Build history of the part. All positions in model axes, mm. A direction names the side the tool comes from. Round coordinates to 2 decimals unless told otherwise and drop trailing zeros. Write each loop counter-clockwise with the first axis right and the second up, starting at its lowest first coordinate (ties: lowest second). Pieces come first, ordered by that corner, then holes. Notation, with made-up numbers: (-1.5, 20) - (27.5, 20) arc R7 cw to (27.5, 33) - close; hole circle Ø7 at (-21, 39.5). An arc over 180 degrees is marked (long way). Answer as a JSON object with one key per item and string values. Group by question number.
Item 1: Which spindle directions (+Z, -Z, +X, -X, +Y, -Y) get a long thin tool onto all of the face, cutting with end or side? Do faces 1 (the flat face through (13.52, 5.77, 41.77)), 2 (the flat face through (7.254, 4.056, -15.687)), 3 (the cylindrical face through (9.31, 7.43, -43.15)). Say none if no direction does.
Item 2: Slice it at D-D, the plane z = -38.75. List the corners of the cut face in (x, y).
Item 3: Two-plate mould, pull along X, no slides. Class faces 4 (the cylindrical face through (9, 4, 41)), 5 (the flat face through (14.3, 7.2, -0.6)), 6 (the flat face through (10.032, 4, 10)), 7 (the flat face through (-14.26, 3.97, -42.99)): +X half, -X half, draft (parallel to the pull), parting line (faces both ways), or undercut.
Item 4: Flat gauge pins, fed straight in: pin 1 (3.5 mm diameter, centred on y = 4, z = 38.75, fed in from -X) (3 decimals); pin 2 (2.5 mm diameter, centred on x = -2.5, y = 5, fed in from +Z). Where does each tip first touch, or does it go through?
Item 5: Probe line 1 (Y direction, x = 8.5, z = -38.75); line 2 (Y direction, x = 12.25, z = 40.5); line 3 (X direction, y = 4.25, z = -13.5). List the from-to ranges inside material, lowest first. Write a range as from..to.
Item 6: Slice it at B-B, the plane x = -7. List the corners of the cut face in (y, z).
Item 7: Slice it at A-A, the plane z = 38.75. List the corners of the cut face in (x, y).
Item 8: Slice it at C-C, the plane x = -12.25. List the corners of the cut face in (y, z).
from build123d import *

# Parameters (mm, degrees)
SKETCH1_W           = 30
SKETCH1_H           = 87.5
BOSS_EXTRUDE1_DEPTH = 8
SKETCH2_W           = 10
SKETCH2_H           = 12
CUT_EXTRUDE1_DEPTH  = 8
SKETCH3_R           = 2.25
CUT_EXTRUDE2_DEPTH  = 54.647576833
FILLET1_R           = 2
CUT_EXTRUDE3_DEPTH  = 47.936792605
FILLET2_R           = 3
CHAMFER1_SIZE       = 1.5
FILLET3_R           = 0.5
CUT_EXTRUDE4_DEPTH  = 3


with BuildPart() as part:
    # Sketch1 → Boss-Extrude1 (new body)
    with BuildSketch(Plane(origin=(0, 0, 0), x_dir=(1, 0, 0), z_dir=(0, 1, 0))):
        Rectangle(SKETCH1_W, SKETCH1_H)
    extrude(amount=BOSS_EXTRUDE1_DEPTH)

    # Sketch2 → Cut-Extrude1 (cut)
    with BuildSketch(Plane(origin=(0, 8, 0), x_dir=(1, 0, 0), z_dir=(0, 1, 0))):
        with Locations((0, 37.75)):
            Rectangle(SKETCH2_W, SKETCH2_H)
        with Locations((0, -37.75)):
            Rectangle(SKETCH2_W, SKETCH2_H)
    extrude(amount=-CUT_EXTRUDE1_DEPTH, mode=Mode.SUBTRACT)

    # Sketch3 → Cut-Extrude2 (cut, through all)
    with BuildSketch(Plane(origin=(15, 0, 0), x_dir=(0, 0, -1), z_dir=(1, 0, 0))):
        with Locations((-38.75, 4)):
            Circle(SKETCH3_R)
    cut_extrude2 = extrude(amount=-CUT_EXTRUDE2_DEPTH, mode=Mode.SUBTRACT)

    # Mirror1: Cut-Extrude2 across plane
    add(cut_extrude2.mirror(Plane.XY), mode=Mode.SUBTRACT)

    # Fillet1
    fillet1_edges = [part.edges().sort_by_distance(p)[0] for p in [
        (10, 0, 43.75),
        (-10, 0, -43.75),
        (-10, 8, 43.75),
        (-10, 8, -43.75),
        (10, 8, 43.75),
        (-10, 0, 43.75),
        (10, 0, -43.75),
        (10, 8, -43.75),
    ]]
    fillet(fillet1_edges, radius=FILLET1_R)

    # Sketch4 → Cut-Extrude3 (cut, through all)
    with BuildSketch(Plane(origin=(0, 8, 0), x_dir=(1, 0, 0), z_dir=(0, 1, 0))):
        Polygon((5, 24.75), (-10, 24.75), (1.511627907, 13.238372093), align=None)
        Polygon((10, 4.75), (10, 24.75), (5.348837209, 9.401162791), align=None)
        Polygon((-10, -4.75), (-10, -24.75), (-5.348837209, -9.401162791), align=None)
        Polygon((-5, -24.75), (10, -24.75), (-1.511627907, -13.238372093), align=None)
        Polygon((-10, 17.678932188), (-10, 2.321067812), (-3.704402834, -3.974529354), (-0.132806468, 7.811738656), align=None)
        Polygon((10.032301404, -17.711233593), (10.032301404, -2.353369216), (3.704402834, 3.974529354), (0.132806468, -7.811738656), align=None)
    extrude(amount=-CUT_EXTRUDE3_DEPTH, mode=Mode.SUBTRACT)

    # Fillet2
    fillet2_edges = [part.edges().sort_by_distance(p)[0] for p in [
        (0, 0, -31.75),
        (0, 0, 31.75),
    ]]
    fillet(fillet2_edges, radius=FILLET2_R)

    # Chamfer1
    chamfer1_edges = [part.edges().sort_by_distance(p)[0] for p in [
        (15, 4, -43.75),
        (15, 0, 0),
        (-15, 0, 0),
        (15, 8, 0),
        (15, 4, 43.75),
        (15, 7.414213562, 43.164213562),
        (15, 0.585786438, 43.164213562),
        (15, 7.414213562, -43.164213562),
        (15, 0.585786438, -43.164213562),
        (-15, 8, 0),
        (-15, 4, 43.75),
        (-15, 4, -43.75),
        (-15, 0.585786438, 43.164213562),
        (-15, 7.414213562, 43.164213562),
        (-15, 0.585786438, -43.164213562),
        (-15, 7.414213562, -43.164213562),
    ]]
    chamfer(chamfer1_edges, length=CHAMFER1_SIZE)

    # Fillet3
    fillet3_edges = [part.edges().sort_by_distance(p)[0] for p in [
        (-10, 4, -17.678932188),
        (-0.132806468, 4, -7.811738656),
        (-3.704402834, 4, 3.974529354),
        (-10, 4, -2.321067812),
        (-1.511627907, 4, 13.238372093),
        (10, 4, 24.75),
        (-5, 4, 24.75),
        (10, 4, -4.75),
        (5.348837209, 4, -9.401162791),
        (10, 4, -24.75),
        (-10, 4, 4.75),
        (-5.348837209, 4, 9.401162791),
        (-10, 4, 24.75),
        (10.032301404, 4, 17.711233593),
        (0.132806468, 4, 7.811738656),
        (3.704402834, 4, -3.974529354),
        (10.032301404, 4, 2.353369216),
        (5, 4, -24.75),
        (1.511627907, 4, -13.238372093),
        (-10, 4, -24.75),
    ]]
    fillet(fillet3_edges, radius=FILLET3_R)

    # Sketch5 → Cut-Extrude4 (cut)
    with BuildSketch(Plane(origin=(15, 0, 0), x_dir=(0, 0, -1), z_dir=(1, 0, 0))):
        Polygon((-34.708548116, 4), (-36.729274058, 7.5), (-40.770725942, 7.5), (-42.791451884, 4), (-40.770725942, 0.5), (-36.729274058, 0.5), align=None)
    extrude(amount=-CUT_EXTRUDE4_DEPTH, mode=Mode.SUBTRACT)


solid = part.part
Geometry says:
{
 "1": {"face 1": "+X", "face 2": "+Y, -Y", "face 3": "-Z, +X, -X, +Y"},
 "2": {"outline": "(-15, 1.5) - (-13.5, 0) - (-5, 0) - (-5, 1.75) - (-15, 1.75) - close; (-15, 6.25) - (-5, 6.25) - (-5, 8) - (-13.5, 8) - (-15, 6.5) - close; (5, 0) - (13.5, 0) - (15, 1.5) - (15, 1.75) - (5, 1.75) - close; (5, 6.25) - (15, 6.25) - (15, 6.5) - (13.5, 8) - (5, 8) - close"},
 "3": {"face 4": "draft", "face 5": "+X half", "face 6": "undercut", "face 7": "-X half"},
 "4": {"pin 1": "passes through", "pin 2": "stops at z = 31.75"},
 "5": {"line 1": "y = 0..1.75, 6.25..8", "line 2": "y = 0..0.5, 7.5..8", "line 3": "x = -15..-10, -5.82..6.59, 10..15"},
 "6": {"outline": "(0, -41.75) arc R2 ccw to (2, -43.75) - (6, -43.75) arc R2 ccw to (8, -41.75) - (8, -24.75) - (0, -24.75) - close; (0, -21.75) - (8, -21.75) - (8, -14.68) - (0, -14.68) - close; (0, 0.68) - (8, 0.68) - (8, 7.75) - (0, 7.75) - close; (0, 14.85) - (8, 14.85) - (8, 41.75) arc R2 ccw to (6, 43.75) - (2, 43.75) arc R2 ccw to (0, 41.75) - close; hole circle Ø4.5 at (4, -38.75); hole circle Ø4.5 at (4, 38.75)"},
 "7": {"outline": "(-15, 1.5) - (-13.5, 0) - (-5, 0) - (-5, 1.75) - (-15, 1.75) - close; (-15, 6.25) - (-5, 6.25) - (-5, 8) - (-13.5, 8) - (-15, 6.5) - close; (5, 0) - (13.5, 0) - (14, 0.5) - (12, 0.5) - (12, 1.75) - (5, 1.75) - close; (5, 6.25) - (12, 6.25) - (12, 7.5) - (14, 7.5) - (13.5, 8) - (5, 8) - close"},
 "8": {"outline": "(0, -41.75) arc R2 ccw to (2, -43.75) - (6, -43.75) arc R2 ccw to (8, -41.75) - (8, 41.75) arc R2 ccw to (6, 43.75) - (2, 43.75) arc R2 ccw to (0, 41.75) - close; hole circle Ø4.5 at (4, -38.75); hole circle Ø4.5 at (4, 38.75)"}
}
